Source: CAD feature listing. Evaluate the final solid. Frame: model axes, mm. Face numbers are marked on the shaded views. Round coordinates to 2 decimals unless told otherwise and drop trailing zeros. Write each loop counter-clockwise with the first axis right and the second up, starting at its lowest first coordinate (ties: lowest second). Pieces come first, ordered by that corner, then holes. Notation, with made-up numbers: (68.5, 24) -> (107.5, 24) arc R25 ccw to (107.5, 40) -> close; hole circle Ø4 at (42, -5). An arc over 180 degrees is marked (long way). Put each result on its own line as item: value.
```python
from build123d import *

# Parameters (mm, degrees)
SHELL1_T                = -1.27
CUT_EXTRUDE1_DEPTH      = 110.742992031
CUT_EXTRUDE1_DEPTH_BACK = 110.742992031
SKETCH3_R               = 1.0795


with BuildPart() as part:
    # Sketch1 → Revolve1 (revolve)
    with BuildSketch(Plane.XY):
        Polygon((-5.517444444, 25.4), (-1.5875, 0), (0, 0), (0, 105.41), (-21.59, 105.41), (-21.59, 29.21), align=None)
    revolve(axis=Axis((0, 105.41, 0), (0, -1, 0)))

    # Shell1
    shell1_openings = [part.faces().sort_by_distance(p)[0] for p in [
        (0, 105.41, 0),
    ]]
    offset(amount=SHELL1_T, openings=shell1_openings, kind=Kind.INTERSECTION)

    # Sketch3 → Cut-Extrude1 (cut, two sides: drawn at the far end of the back side and taken through both)
    with BuildSketch(Plane.XZ.offset(-CUT_EXTRUDE1_DEPTH_BACK)):
        Circle(SKETCH3_R)
    extrude(amount=CUT_EXTRUDE1_DEPTH + CUT_EXTRUDE1_DEPTH_BACK, mode=Mode.SUBTRACT)


solid = part.part
```
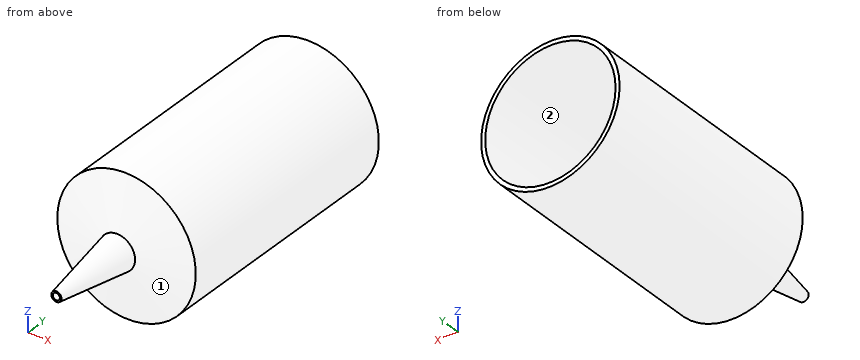
Q1. Cut plane B-B on x = 0. Output: boundary loops of the cut face in (y, z), and give its area (3 significant figures).
Ans:
outline: (0, -1.59) -> (25.4, -5.52) -> (29.21, -21.59) -> (105.41, -21.59) -> (105.41, -20.32) -> (30.21, -20.32) -> (26.44, -4.39) -> (5.02, -1.08) -> (0, -1.08) -> close; (0, 1.08) -> (5.02, 1.08) -> (26.44, 4.39) -> (30.21, 20.32) -> (105.41, 20.32) -> (105.41, 21.59) -> (29.21, 21.59) -> (25.4, 5.52) -> (0, 1.59) -> close
area: 297 mm^2
Q2. Draft query along Z for the marked faces 1 and 2. Return one class per face: +Z half, -Z half, draft (parallel to the pull), parting line (faces both ways), or undercut.
Ans:
face 1: parting line
face 2: undercut
Q3. Cut plane A-A on z = 0. Output: boundary loops of the cut face in (x, y).
Ans:
outline: (-21.59, 29.21) -> (-5.52, 25.4) -> (-1.59, 0) -> (-1.08, 0) -> (-1.08, 5.02) -> (-4.39, 26.44) -> (-20.32, 30.21) -> (-20.32, 105.41) -> (-21.59, 105.41) -> close; (1.08, 0) -> (1.59, 0) -> (5.52, 25.4) -> (21.59, 29.21) -> (21.59, 105.41) -> (20.32, 105.41) -> (20.32, 30.21) -> (4.39, 26.44) -> (1.08, 5.02) -> close
Q4. Material intervals for line 1 (Z direction, x = -0.5, y = 51); line 2 (X direction, y = 62, z = 0); line 3 (X direction, y = 85, z = 1.5), sorted ascending. Write a range as [from, to].
Ans:
line 1: z = [-21.58, -20.31], [20.31, 21.58]
line 2: x = [-21.59, -20.32], [20.32, 21.59]
line 3: x = [-21.54, -20.26], [20.26, 21.54]
Q5. Cut plane C-C on y = 45.5. Output: boundary loops of the cut face in (x, z).
Ans:
outline: circle Ø43.18 at (0, 0); hole circle Ø40.64 at (0, 0)
Q6. Cut plane D-D on y = 14. Output: boundary loops of the cut face in (x, z).
Ans:
outline: circle Ø7.51 at (0, 0); hole circle Ø4.94 at (0, 0)
Q7. Pin query (flat end, axial travel): pin 1 (5 mm diameter, centred on x = -0.5, y = 87.5, fed in from +Z); pin 2 (1.5 mm diameter, centred on x = 0, y = 17, fed in from -Z); pin 3 (8 mm diameter, centred on x = -7.5, z = 17, fed in from -Y). Return the tip coordinate at first contact, or that it passes through.
Ans:
pin 1: stops at z = 21.59
pin 2: stops at z = -4.33
pin 3: stops at y = 27.55
